CAD build for the part. Positions are in the model's coordinates, mm. A direction names the side the tool comes from. Coordinates: 2 decimals unless noted, no trailing zeros. Order: outer loops, then holes, each group sorted by start corner. A loop starts at its lowest first (then second) coordinate and runs counter-clockwise, first axis right, second up. Notation, with made-up numbers: M 12,-4.5 L 28,-4.5 A22 cw 28,12.5 Z; hole C -9.5,73.25 d2. An arc over 180 degrees is marked long. One line per item, written item: value.
from build123d import *

# Parameters (mm, degrees)
SKETCH_1_W          = 55
SKETCH_1_H          = 129
SKETCH_1_W_2        = 30
SKETCH_1_H_2        = 6
EXTRUDE_1_DEPTH     = 3
SKETCH_2_R          = 1.75
CUT_EXTRUDE_1_DEPTH = 10
SKETCH_3_R          = 1.75
CUT_EXTRUDE_2_DEPTH = 10
CHAMFER_1_SIZE      = 2
CHAMFER_2_SIZE      = 2
CUT_EXTRUDE_3_DEPTH = 3
CUT_EXTRUDE_4_DEPTH = 10
FILLET_1_R          = 3
FILLET_2_R          = 3


with BuildPart() as part:
    # Эскиз1 → Бобышка-Вытянуть1 (new body)
    with BuildSketch(Plane.XY):
        Rectangle(SKETCH_1_W, SKETCH_1_H)
        with Locations((0, 64.5)):
            Rectangle(SKETCH_1_W_2, SKETCH_1_H_2)
        with Locations((0, -64.5)):
            Rectangle(SKETCH_1_W_2, SKETCH_1_H_2)
    extrude(amount=EXTRUDE_1_DEPTH)

    # Эскиз2 → Вырез-Вытянуть1 (cut)
    with BuildSketch(Plane.XY.offset(3)):
        with Locations((-15.35, 45.7)):
            Circle(SKETCH_2_R)
        with Locations((15.35, 45.7)):
            Circle(SKETCH_2_R)
        with Locations((15.35, 15)):
            Circle(SKETCH_2_R)
        with Locations((-15.35, 15)):
            Circle(SKETCH_2_R)
        with Locations((-15.35, -15)):
            Circle(SKETCH_2_R)
        with Locations((15.35, -15)):
            Circle(SKETCH_2_R)
        with Locations((15.35, -45.7)):
            Circle(SKETCH_2_R)
        with Locations((-15.35, -45.7)):
            Circle(SKETCH_2_R)
    extrude(amount=-CUT_EXTRUDE_1_DEPTH, mode=Mode.SUBTRACT)

    # Эскиз3 → Вырез-Вытянуть2 (cut)
    with BuildSketch(Plane(origin=(0, 0, 0), x_dir=(-1, 0, 0), z_dir=(0, 0, -1))):
        with Locations((-22.5, 30.35)):
            Circle(SKETCH_3_R)
        with Locations((-12.5, 30.35)):
            Circle(SKETCH_3_R)
        with Locations((-5, 30.35)):
            Circle(SKETCH_3_R)
        with Locations((5, 30.35)):
            Circle(SKETCH_3_R)
        with Locations((12.5, 30.35)):
            Circle(SKETCH_3_R)
        with Locations((22.5, 30.35)):
            Circle(SKETCH_3_R)
        with Locations(Location((22.5, -30.35, 0), (0, 0, 180))):
            Circle(SKETCH_3_R)
        with Locations(Location((12.5, -30.35, 0), (0, 0, 180))):
            Circle(SKETCH_3_R)
        with Locations(Location((5, -30.35, 0), (0, 0, 180))):
            Circle(SKETCH_3_R)
        with Locations(Location((-5, -30.35, 0), (0, 0, 180))):
            Circle(SKETCH_3_R)
        with Locations(Location((-12.5, -30.35, 0), (0, 0, 180))):
            Circle(SKETCH_3_R)
        with Locations(Location((-22.5, -30.35, 0), (0, 0, 180))):
            Circle(SKETCH_3_R)
    extrude(amount=-CUT_EXTRUDE_2_DEPTH, mode=Mode.SUBTRACT)

    # Фаска1
    chamfer_1_edges = [part.edges().sort_by_distance(p)[0] for p in [
        (-17.1, -15, 0),
        (-17.1, 15, 0),
        (13.6, 15, 0),
        (-17.1, 45.7, 0),
        (13.6, -15, 0),
        (13.6, -45.7, 0),
        (-17.1, -45.7, 0),
        (13.6, 45.7, 0),
    ]]
    chamfer(chamfer_1_edges, length=CHAMFER_1_SIZE)

    # Фаска2
    chamfer_2_edges = [part.edges().sort_by_distance(p)[0] for p in [
        (-6.75, -30.35, 3),
        (-14.25, -30.35, 3),
        (-24.25, -30.35, 3),
        (-20.75, 30.35, 3),
        (-10.75, 30.35, 3),
        (-3.25, 30.35, 3),
        (6.75, 30.35, 3),
        (14.25, 30.35, 3),
        (3.25, -30.35, 3),
        (10.75, -30.35, 3),
        (20.75, -30.35, 3),
        (24.25, 30.35, 3),
    ]]
    chamfer(chamfer_2_edges, length=CHAMFER_2_SIZE - 0.0001)  # a hair under: the kernel refuses the full size

    # Эскиз4 → Вырез-Вытянуть3 (cut)
    with BuildSketch(Plane(origin=(0, 0, 0), x_dir=(-1, 0, 0), z_dir=(0, 0, -1))):
        Polygon((7.5, 11.25), (-7.5, 11.25), (-13.75, 5), (-13.75, -5), (-7.5, -11.25), (7.5, -11.25), (13.75, -5), (13.75, 5), align=None)
    extrude(amount=-CUT_EXTRUDE_3_DEPTH, mode=Mode.SUBTRACT)

    # Эскиз6 → Вырез-Вытянуть4 (cut)
    with BuildSketch(Plane.XY.offset(3)):
        Polygon((21.25, 64.5), (21.25, 51.75), (27.5, 45.5), (29.222592787, 45.5), (29.222592787, 64.5), align=None)
        Polygon((-29.222592787, 45.5), (-27.5, 45.5), (-21.25, 51.75), (-21.25, 64.5), (-29.222592787, 64.5), align=None)
        Polygon((-21.25, -64.5), (-21.25, -51.75), (-27.5, -45.5), (-29.222592787, -45.5), (-29.222592787, -64.5), align=None)
        Polygon((29.222592787, -45.5), (27.5, -45.5), (21.25, -51.75), (21.25, -64.5), (29.222592787, -64.5), align=None)
        Polygon((-27.5, 18.35), (-21.25, 12.1), (-21.25, -12.1), (-27.5, -18.35), (-29.834520007, -18.35), (-29.834520007, 18.35), align=None)
        Polygon((27.5, -18.35), (21.25, -12.1), (21.25, 12.1), (27.5, 18.35), (30.388553895, 18.35), (30.388553895, -18.35), align=None)
    extrude(amount=-CUT_EXTRUDE_4_DEPTH, mode=Mode.SUBTRACT)

    # Скругление1
    fillet_1_edges = [part.edges().sort_by_distance(p)[0] for p in [
        (-27.5, 18.35, 1.5),
        (-21.25, 12.1, 1.5),
        (-21.25, -12.1, 1.5),
        (-27.5, -18.35, 1.5),
        (21.25, -51.75, 1.5),
        (27.5, -45.5, 1.5),
        (-27.5, -45.5, 1.5),
        (-21.25, -51.75, 1.5),
        (-21.25, 51.75, 1.5),
        (-27.5, 45.5, 1.5),
        (27.5, -18.35, 1.5),
        (21.25, -12.1, 1.5),
        (21.25, 12.1, 1.5),
        (27.5, 18.35, 1.5),
        (27.5, 45.5, 1.5),
        (21.25, 51.75, 1.5),
    ]]
    fillet(fillet_1_edges, radius=FILLET_1_R)

    # Скругление2
    fillet_2_edges = [part.edges().sort_by_distance(p)[0] for p in [
        (-7.5, -11.25, 1.5),
        (7.5, -11.25, 1.5),
        (13.75, -5, 1.5),
        (13.75, 5, 1.5),
        (7.5, 11.25, 1.5),
        (-7.5, 11.25, 1.5),
        (-13.75, 5, 1.5),
        (-13.75, -5, 1.5),
    ]]
    fillet(fillet_2_edges, radius=FILLET_2_R)


solid = part.part
Q1. Pin check, flat tips, straight feed: pin 1 Ø0.9 at (y, z) = (-60.5, 2) entering from +X; pin 2 Ø0.9 at (y, z) = (5, 1) entering from -X; pin 3 Ø0.9 at (y, z) = (-66.5, 1.5) entering from +X. Stop position of each tip, or through.
Recorded:
pin 1: stops at x = 21.25
pin 2: stops at x = -21.25
pin 3: stops at x = 15
Q2. Mould opens along X. For faces 3 (the face through (-11.69, -28.8, 0.49)), 4 (the face through (24.41, -15.26, 1.52)), 5 (the face through (-24, 49, 2)), 6 (the face through (0, 16, 3)) say: released by +X, released by -X, zero draft, split by the parting line, or undercut.
Recorded:
face 3: undercut
face 4: released by +X
face 5: released by -X
face 6: zero draft
Q3. Slice it at C-C (z = 0.5). Give the number of separate pieces and of enclosed holes in the cut face, plus the area to 3 significant figures.
Recorded:
separate pieces: 1
enclosed holes: 21
area: 5,580 mm^2
Q4. Slice it at B-B (y = -55.5). List the corners of the cut face in (x, z), plus the area to 4 significant figures.
Recorded:
outline: M -21.25,0 L 21.25,0 L 21.25,3 L -21.25,3 Z
area: 127.5 mm^2
Q5. Which spindle directions (+Z, -Z, +X, -X, +Y, -Y) get a long thin tool onto all of the face, cutting with end or side? Do faces 1 (the face through (-15.578, 47.435, 2.507)), 2 (the face through (18, -64.5, 1)). Say none if no direction does.
Recorded:
face 1: +Z, -Z
face 2: +Z, -Z, +X, -Y
Q6. Slice it at A-A (x = 5). List the corners of the cut face in (y, z).
Recorded:
outline: M -67.5,0 L -32.1,0 L -32.1,1 L -34.1,3 L -67.5,3 Z; M -28.6,0 L -11.25,0 L -11.25,3 L -26.6,3 L -28.6,1 Z; M 11.25,0 L 28.6,0 L 28.6,1 L 26.6,3 L 11.25,3 Z; M 32.1,0 L 67.5,0 L 67.5,3 L 34.1,3 L 32.1,1 Z
Q7. Drill centre lines: line 1 along Y through (x, z) = (5, 0.75); line 2 along Y through (x, z) = (-4, 0.4); line 3 along Y through (x, z) = (17, 1.2). Where is each one in solid material? Low to high.
Recorded:
line 1: y = -67.5 to -32.1, -28.6 to -11.25, 11.25 to 28.6, 32.1 to 67.5
line 2: y = -67.5 to -31.79, -28.91 to -11.25, 11.25 to 28.91, 31.79 to 67.5
line 3: y = -64.5 to -47.64, -43.76 to -16.94, -13.06 to 13.06, 16.94 to 43.76, 47.64 to 64.5
